Work out the finished part from the listing and answer in its coordinate system (mm). Face numbers are marked on the shaded views. A direction names the side the tool comes from. Round coordinates to 2 decimals unless told otherwise and drop trailing zeros. Loops run counter-clockwise (first coordinate to the right, second up) from the corner with the lowest first, then second, coordinate; pieces in that order, holes last. Notation, with made-up numbers: (62, 44) -> (88, 44) arc R12 cw to (88, 48) -> close; hole circle Ø6 at (49, 56). An arc over 180 degrees is marked (long way). Use CSV: the item, a comma, the result in double quotes. Start each with the question number.
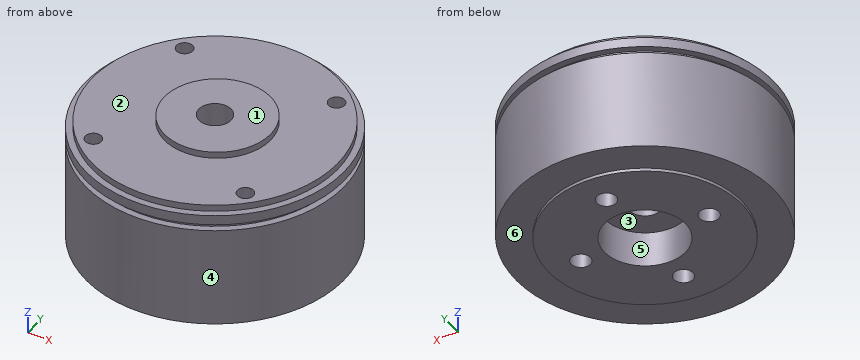
from build123d import *

# Parameters (mm, degrees)
SKETCH_1_R               = 20
EXTRUDE_1_DEPTH          = 20
SKETCH_2_R               = 15
EXTRUDE_2_DEPTH          = 0.5
CUT_EXTRUDE_2_DEPTH      = 4
CUT_EXTRUDE_2_DEPTH_BACK = 4
SKETCH_3_R               = 1.5
CUT_EXTRUDE_START        = -1
SKETCH_4_R               = 20
SKETCH_4_R_2             = 8.25
CUT_EXTRUDE_3_DEPTH      = 1
CUT_EXTRUDE_START_2      = -2
SKETCH_5_R               = 20
SKETCH_5_R_2             = 19
CUT_EXTRUDE_4_DEPTH      = 2
SKETCH_6_R               = 20
SKETCH_6_R_2             = 19
CUT_EXTRUDE_5_DEPTH      = 1
SKETCH_7_R               = 1.25
CUT_EXTRUDE_6_DEPTH      = 5
CUT_EXTRUDE_7_DEPTH      = 5
CUT_EXTRUDE_7_DEPTH_BACK = 35.641016151
SKETCH_8_R               = 6.3
CUT_EXTRUDE_8_DEPTH      = 35.641016151
CUT_EXTRUDE_8_DEPTH_BACK = 35.641016151
SKETCH_9_R               = 2.5


with BuildPart() as part:
    # 草图1 → 凸台-拉伸1 (new body)
    with BuildSketch(Plane.XY):
        Circle(SKETCH_1_R)
    extrude(amount=EXTRUDE_1_DEPTH)

    # 草图2 → 凸台-拉伸2 (add)
    with BuildSketch(Plane.XY):
        Circle(SKETCH_2_R)
    extrude(amount=-EXTRUDE_2_DEPTH)

    # 草图3 → 切除-拉伸2 (cut, two sides: drawn at the far end of the back side and taken through both)
    with BuildSketch(Plane.XY.offset(-CUT_EXTRUDE_2_DEPTH_BACK)):
        with Locations((0, 10)):
            Circle(SKETCH_3_R)
        with Locations((10, 0)):
            Circle(SKETCH_3_R)
        with Locations((0, -10)):
            Circle(SKETCH_3_R)
        with Locations((-10, 0)):
            Circle(SKETCH_3_R)
    extrude(amount=CUT_EXTRUDE_2_DEPTH + CUT_EXTRUDE_2_DEPTH_BACK, mode=Mode.SUBTRACT)

    # 草图4 → 切除-拉伸3 (cut)
    with BuildSketch(Plane.XY.offset(20).offset(CUT_EXTRUDE_START)):
        Circle(SKETCH_4_R)
        with Locations((0.385039993, 0)):
            Circle(SKETCH_4_R_2, mode=Mode.SUBTRACT)
    extrude(amount=CUT_EXTRUDE_3_DEPTH, mode=Mode.SUBTRACT)

    # 草图5 → 切除-拉伸4 (cut)
    with BuildSketch(Plane.XY.offset(20).offset(CUT_EXTRUDE_START_2)):
        Circle(SKETCH_5_R)
        Circle(SKETCH_5_R_2, mode=Mode.SUBTRACT)
    extrude(amount=CUT_EXTRUDE_4_DEPTH, mode=Mode.SUBTRACT)

    # 草图6 → 切除-拉伸5 (cut)
    with BuildSketch(Plane.XY.offset(16.5).offset(CUT_EXTRUDE_START)):
        Circle(SKETCH_6_R)
        Circle(SKETCH_6_R_2, mode=Mode.SUBTRACT)
    extrude(amount=CUT_EXTRUDE_5_DEPTH, mode=Mode.SUBTRACT)

    # 草图7 → 切除-拉伸6 (cut)
    with BuildSketch(Plane.XY.offset(20)):
        with Locations((-11.844038585, -11.844038585)):
            Circle(SKETCH_7_R)
        with Locations((-11.844038585, 11.844038585)):
            Circle(SKETCH_7_R)
        with Locations((11.844038585, 11.844038585)):
            Circle(SKETCH_7_R)
        with Locations((11.844038585, -11.844038585)):
            Circle(SKETCH_7_R)
    extrude(amount=-CUT_EXTRUDE_6_DEPTH, mode=Mode.SUBTRACT)

    # 草图8 → 切除-拉伸7 (cut, two sides: drawn at the far end of the back side and taken through both)
    with BuildSketch(Plane.XY.offset(-CUT_EXTRUDE_7_DEPTH_BACK)):
        Circle(SKETCH_8_R)
    extrude(amount=CUT_EXTRUDE_7_DEPTH + CUT_EXTRUDE_7_DEPTH_BACK, mode=Mode.SUBTRACT)

    # 草图9 → 切除-拉伸8 (cut, two sides: drawn at the far end of the back side and taken through both)
    with BuildSketch(Plane.XY.offset(-CUT_EXTRUDE_8_DEPTH_BACK)):
        Circle(SKETCH_9_R)
    extrude(amount=CUT_EXTRUDE_8_DEPTH + CUT_EXTRUDE_8_DEPTH_BACK, mode=Mode.SUBTRACT)


solid = part.part
Q1. Section A-A, the plane z = 4.5 is taken. Write down the section's boundary in (x, y), and give its area (3 significant figures).
Q2. Section B-B, the plane x = 4 is taken. Write down the section's boundary in (y, z), and give its area (3 significant figures).
Q3. Straight lines are drawn through the part: line 1 (Z direction, x = -14, y = -14); line 2 (Y direction, x = 0, z = 1.55); line 3 (Y direction, x = 0, z = 11.5). For each, find the intervals that lie inside material, in ascending order. Write a range as from..to.
Q4. Which of the six approach directions +Z, -Z, +X, -X, +Y, -Y give full straight-line access (tool end or side, diameter ignored) to the marked faces 1, 2 and 3?
Q5. For a pull along Y with two mould halves and no side action, classify the marked faces 4, 5 and 6 as pulls with the +Y half, pulls with the -Y half, needs draft (parallel to the pull), parting line crosses it, or undercut.
Q6. Section D-D, the plane y = 18 is taken. Write down the section's boundary in (x, z), and give its area (3 significant figures).
Q7. Each of these flat-tipped pins is pushed along its axis until it touches: pin 1 (2.5 mm diameter, centred on x = -10, y = 0, fed in from -Z); pin 2 (1.5 mm diameter, centred on x = 3.5, y = -12.5, fed in from +Z); pin 3 (10 mm diameter, centred on x = 9.5, z = 4, fed in from +Y). Where does it stop, or does it pass through?
Q8. Section C-C, the plane y = -9 is taken. Write down the section's boundary in (x, z), and give its area (3 significant figures).
Report:
1,outline,"circle Ø40 at (0, 0); hole circle Ø12.6 at (0, 0)"
1,area,"1,130 mm²"
2,outline,"(-19.6, 0) -> (-14.46, 0) -> (-14.46, -0.5) -> (-4.87, -0.5) -> (-4.87, 5) -> (4.87, 5) -> (4.87, -0.5) -> (14.46, -0.5) -> (14.46, 0) -> (19.6, 0) -> (19.6, 15.5) -> (18.57, 15.5) -> (18.57, 16.5) -> (19.6, 16.5) -> (19.6, 18) -> (18.57, 18) -> (18.57, 19) -> (7.42, 19) -> (7.42, 20) -> (-7.42, 20) -> (-7.42, 19) -> (-18.57, 19) -> (-18.57, 18) -> (-19.6, 18) -> (-19.6, 16.5) -> (-18.57, 16.5) -> (-18.57, 15.5) -> (-19.6, 15.5) -> close"
2,area,"716 mm²"
3,line 1,"z = 0..15.5, 16.5..18"
3,line 2,"y = -20..-11.5, -8.5..-6.3, 6.3..8.5, 11.5..20"
3,line 3,"y = -20..-2.5, 2.5..20"
4,face 1,"+Z, +X, -X, +Y, -Y"
4,face 2,"+Z"
4,face 3,"-Z"
5,face 4,"parting line crosses it"
5,face 5,"undercut"
5,face 6,"needs draft"
6,outline,"(-8.72, 0) -> (8.72, 0) -> (8.72, 15.5) -> (6.08, 15.5) -> (6.08, 16.5) -> (8.72, 16.5) -> (8.72, 18) -> (6.08, 18) -> (6.08, 19) -> (-6.08, 19) -> (-6.08, 18) -> (-8.72, 18) -> (-8.72, 16.5) -> (-6.08, 16.5) -> (-6.08, 15.5) -> (-8.72, 15.5) -> close"
6,area,"321 mm²"
7,pin 1,"stops at z = 4"
7,pin 2,"stops at z = 19"
7,pin 3,"stops at y = 19.49"
8,outline,"(-17.86, 0) -> (-12, 0) -> (-12, -0.5) -> (-1.12, -0.5) -> (-1.12, 4) -> (1.12, 4) -> (1.12, -0.5) -> (12, -0.5) -> (12, 0) -> (17.86, 0) -> (17.86, 15.5) -> (16.73, 15.5) -> (16.73, 16.5) -> (17.86, 16.5) -> (17.86, 18) -> (16.73, 18) -> (16.73, 19) -> (-16.73, 19) -> (-16.73, 18) -> (-17.86, 18) -> (-17.86, 16.5) -> (-16.73, 16.5) -> (-16.73, 15.5) -> (-17.86, 15.5) -> close"
8,area,"676 mm²"
